Here's how the part is built. I have some questions about the finished solid (model axes, mm). Face numbers are marked on the shaded views. A direction names the side the tool comes from. Coordinates: 2 decimals unless noted, no trailing zeros. Write each loop counter-clockwise with the first axis right and the second up, starting at its lowest first coordinate (ties: lowest second). Pieces come first, ordered by that corner, then holes. Notation, with made-up numbers: (54.25, 56.25) -> (96.25, 56.25) arc R20 cw to (96.25, 75.25) -> close; hole circle Ø3 at (2.25, 39.25). An arc over 180 degrees is marked (long way). Put each result on its own line as item: value. Start each with the question number.
Item 1: For pin 1 (2 mm diameter, centred on y = 34, z = -16.5, fed in from -X); pin 2 (1 mm diameter, centred on y = 39.5, z = -13, fed in from +X); pin 3 (3 mm diameter, centred on y = 4.5, z = -4, fed in from -X); pin 4 (1.5 mm diameter, centred on x = -2, z = -24, fed in from -Y), each with a flat end and sliding along its axis, tell me the tip position at first contact or that it passes through.
Item 2: If we mould it in two halves opening along Z, with no side actions, what happens to the marked faces 3, 4, 5 and 6? For each: released by +Z, released by -Z, zero draft, split by the parting line, or undercut.
Item 3: I need wall thicknesses on line 1 (Z direction, x = -31.5, y = 4.5); line 2 (Z direction, x = -17, y = 28.5); line 3 (X direction, y = 23.5, z = 7.5). Which ranges of each line are inside material? Lowest first, please. Write a range as [from, to].
Item 4: I want a section at C-C, the plane y = 24. State how many separate pieces and enclosed holes the cut face has, then the cut area to 3 significant figures.
Item 5: I want a section at B-B, the plane z = 15.5. List the corners of the cut face in (x, y) for me.
Item 6: I want a section at A-A, the plane z = 7.5. List the corners of the cut face in (x, y) for me.
Item 7: On a 3-axis mill with a long thin cutter (end or side, diameter ignored), from which of +Z, -Z, +X, -X, +Y, -Y can I reach the whole of each face in a straight line? I mean the marked faces 1 and 2. Say none if no direction works.
Item 8: I want a section at D-D, the plane x = 31.5. List the corners of the cut face in (y, z) for me.
from build123d import *

# Parameters (mm, degrees)
SKETCH1_W           = 127
SKETCH1_H           = 61.9252
BOSS_EXTRUDE1_DEPTH = 44.45
SKETCH1_3_W         = 127
SKETCH1_3_H         = 1.8415
CUT_EXTRUDE2_DEPTH  = 38.1
SKETCH2_W           = 71.12
SKETCH2_H           = 32.258
SKETCH2_W_2         = 35.442647017
SKETCH2_H_2         = 23.182829488
CUT_EXTRUDE3_DEPTH  = 38.1
CHAMFER2_SIZE       = 10.16
CUT_EXTRUDE5_DEPTH  = 100.210800294
FILLET3_R           = 2.54
SKETCH2_3_W         = 35.442647017
SKETCH2_3_H         = 23.182829488
CUT_EXTRUDE6_DEPTH  = 84.466970107
CHAMFER3_SIZE       = 2.54
SKETCH9_W           = 74.62
SKETCH9_H           = 35.758
CUT_EXTRUDE7_DEPTH  = 38.1


with BuildPart() as part:
    # Sketch1 → Boss-Extrude1 (new body)
    with BuildSketch(Plane(origin=(0, 0, 0), x_dir=(1, 0, 0), z_dir=(0, 1, 0))):
        Rectangle(SKETCH1_W, SKETCH1_H)
    extrude(amount=BOSS_EXTRUDE1_DEPTH)

    # Sketch1<3> → Cut-Extrude2 (cut)
    with BuildSketch(Plane(origin=(0, 0, 0), x_dir=(1, 0, 0), z_dir=(0, 1, 0))):
        with Locations((0, 23.69185)):
            Rectangle(SKETCH1_3_W, SKETCH1_3_H)
        with Locations((0, -23.69185)):
            Rectangle(SKETCH1_3_W, SKETCH1_3_H)
    extrude(amount=CUT_EXTRUDE2_DEPTH, mode=Mode.SUBTRACT)

    # Sketch2 → Cut-Extrude3 (cut)
    with BuildSketch(Plane(origin=(0, 44.45, 0), x_dir=(1, 0, 0), z_dir=(0, 1, 0))):
        with Locations((1.016, 0)):
            Rectangle(SKETCH2_W, SKETCH2_H)
        with Locations((12.504676492, 0)):
            Rectangle(SKETCH2_W_2, SKETCH2_H_2, mode=Mode.SUBTRACT)
    extrude(amount=-CUT_EXTRUDE3_DEPTH, mode=Mode.SUBTRACT)

    # Chamfer2
    chamfer2_edges = [part.edges().sort_by_distance(p)[0] for p in [
        (36.576, 44.45, 0),
        (1.016, 44.45, -16.129),
        (-34.544, 44.45, 0),
        (1.016, 44.45, 16.129),
    ]]
    chamfer(chamfer2_edges, length=CHAMFER2_SIZE)

    # Sketch7 → Cut-Extrude5 (cut, through all)
    with BuildSketch(Plane.XY.offset(30.9626)):
        Polygon((-50.795476794, 0), (-63.5, 44.45), (-63.5, 0), align=None)
        Polygon((63.5, 44.45), (50.795476794, 0), (63.5, 0), align=None)
    extrude(amount=-CUT_EXTRUDE5_DEPTH, mode=Mode.SUBTRACT)

    # Fillet3
    fillet3_edges = [part.edges().sort_by_distance(p)[0] for p in [
        (-57.147738397, 22.225, -30.9626),
        (-57.147738397, 22.225, 30.9626),
        (57.147738397, 22.225, 30.9626),
        (57.147738397, 22.225, -30.9626),
    ]]
    fillet(fillet3_edges, radius=FILLET3_R)

    # Sketch2<3> → Cut-Extrude6 (cut, through all)
    with BuildSketch(Plane(origin=(0, 44.45, 0), x_dir=(1, 0, 0), z_dir=(0, 1, 0))):
        with Locations((12.504676492, 0)):
            Rectangle(SKETCH2_3_W, SKETCH2_3_H)
    extrude(amount=-CUT_EXTRUDE6_DEPTH, mode=Mode.SUBTRACT)

    # Chamfer3
    chamfer3_edges = [part.edges().sort_by_distance(p)[0] for p in [
        (30.226, 0, 0),
        (12.504676491, 0, 11.591414744),
        (-5.216647017, 0, 0),
        (12.504676491, 0, -11.591414744),
    ]]
    chamfer(chamfer3_edges, length=CHAMFER3_SIZE)

    # Sketch9 → Cut-Extrude7 (cut)
    with BuildSketch(Plane(origin=(0, 44.45, 0), x_dir=(1, 0, 0), z_dir=(0, 1, 0))):
        with Locations((1.016, 0)):
            Rectangle(SKETCH9_W, SKETCH9_H)
    extrude(amount=-CUT_EXTRUDE7_DEPTH, mode=Mode.SUBTRACT)


solid = part.part
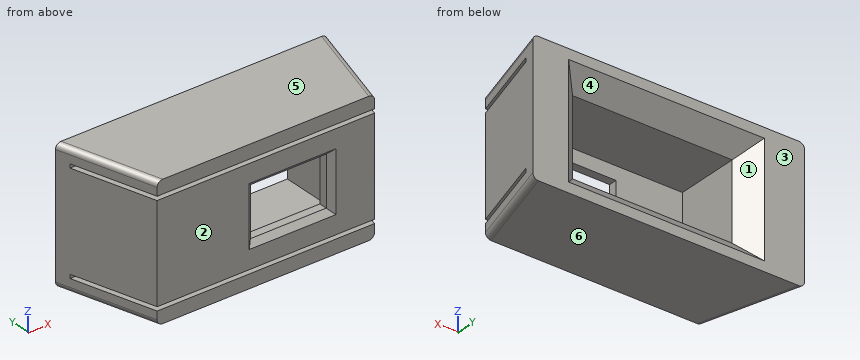
Calculated:
1. pin 1: stops at x = -60.8
1. pin 2: stops at x = 62.23
1. pin 3: stops at x = -52.51
1. pin 4: stops at y = 0
2. face 3: zero draft
2. face 4: undercut
2. face 5: released by +Z
2. face 6: released by -Z
3. line 1: z = [-30.96, -24.61], [-22.77, 22.77], [24.61, 30.96]
3. line 2: z = [-30.96, -24.61], [-22.77, -17.88], [17.88, 22.77], [24.61, 30.96]
3. line 3: x = [-57.51, -36.29], [38.33, 57.51]
4. separate pieces: 3
4. enclosed holes: 1
4. area: 4,040 mm2
5. outline: (-63.5, 44.45) -> (-50.8, 0) -> (50.8, 0) -> (63.5, 44.45) -> (46.74, 44.45) -> (38.33, 36.04) -> (38.33, 6.35) -> (-36.29, 6.35) -> (-36.29, 36.04) -> (-44.7, 44.45) -> close
6. outline: (-63.5, 44.45) -> (-50.8, 0) -> (-7.76, 0) -> (-5.22, 2.54) -> (-5.22, 6.35) -> (-36.29, 6.35) -> (-36.29, 36.04) -> (-44.7, 44.45) -> close; (30.23, 2.54) -> (32.77, 0) -> (50.8, 0) -> (63.5, 44.45) -> (46.74, 44.45) -> (38.33, 36.04) -> (38.33, 6.35) -> (30.23, 6.35) -> close
7. face 1: +Y
7. face 2: +Z, -Z, +X, -X, -Y
8. outline: (0, -30.96) -> (44.45, -30.96) -> (44.45, -26.29) -> (36.04, -17.88) -> (6.35, -17.88) -> (6.35, 17.88) -> (36.04, 17.88) -> (44.45, 26.29) -> (44.45, 30.96) -> (0, 30.96) -> (0, 24.61) -> (38.1, 24.61) -> (38.1, 22.77) -> (0, 22.77) -> (0, 14.13) -> (1.27, 12.87) -> (1.27, -12.87) -> (0, -14.13) -> (0, -22.77) -> (38.1, -22.77) -> (38.1, -24.61) -> (0, -24.61) -> close
